```python
from build123d import *

# Parameters (mm, degrees)
F0_W     = 40
F0_H     = 40
F1_DEPTH = 5
F2_R     = 2
F3_DEPTH = 5
F4_R     = 3
F5_DEPTH = 3


with BuildPart() as f1:
    # F0 (on Top) → F1 (new body)
    with BuildSketch(Plane.XY):
        Rectangle(F0_W, F0_H)
    extrude(amount=F1_DEPTH)

    # F2 (on face) → F3 (cut)
    with BuildSketch(Plane.XY.offset(5)):
        with Locations((-12.70971, -8.583505)):
            Circle(F2_R)
        with Locations((-13.331592, 11.416495)):
            Circle(F2_R)
        with Locations((12.668408, 12.357356)):
            Circle(F2_R)
        with Locations((13.29029, -7.642644)):
            Circle(F2_R)
    extrude(amount=-F3_DEPTH, mode=Mode.SUBTRACT)

    # F4 (on face) → F5 (cut)
    with BuildSketch(Plane.XY.offset(5)):
        with Locations((-12.70971, -8.583505)):
            Circle(F4_R)
        with Locations((-13.331592, 11.416495)):
            Circle(F4_R)
        with Locations((12.668408, 12.357356)):
            Circle(F4_R)
        with Locations((13.29029, -7.642644)):
            Circle(F4_R)
    extrude(amount=-F5_DEPTH, mode=Mode.SUBTRACT)


solid = f1.part
```
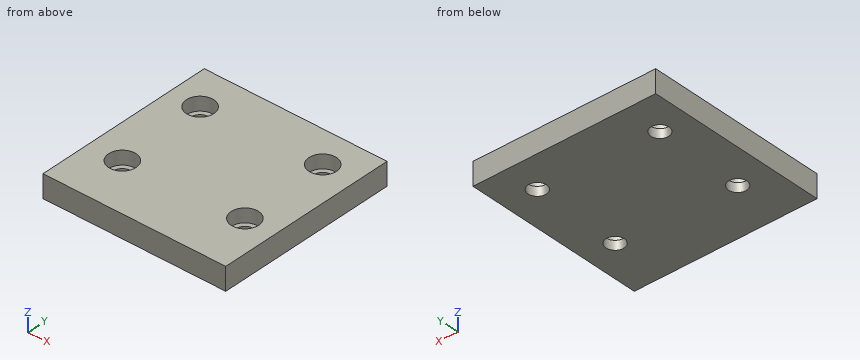
The listing builds one solid part. Answer for the finished solid, in the listing's coordinates (mm). Coordinates: 2 decimals unless noted, no trailing zeros. Loops run counter-clockwise (first coordinate to the right, second up) from the corner with the lowest first, then second, coordinate; pieces in that order, holes last. Notation, with made-up numbers: (57, -13) -> (85, -13) arc R12 cw to (85, -5) -> close; hole circle Ø8 at (61.5, -4). An arc over 180 degrees is marked (long way). Use one line per item in the form item = value. Start each with the question number.
Item 1: The part is cut by section B-B on z = 3. Determine the outline of the cut face in (x, y).
Item 2: A flat-ended cylindrical pin translates along its axis: pin 1 Ø5.5 at (x, y) = (12.67, 12.36) entering from +Z. Find the tip coordinate at first contact, or state that the pin passes through.
Item 3: The part is cut by section D-D on z = 0.55. Determine the outline of the cut face in (x, y), then the cut area to 3 significant figures.
Item 4: The part is cut by section A-A on x = 12. Determine the outline of the cut face in (y, z), then the cut area to 3 significant figures.
Item 5: The part is cut by section C-C on x = -12. Determine the outline of the cut face in (y, z).
Item 6: Consider L1, parallel to Y at x = -11, z = 3.5; L2, parallel to Y at x = 13, z = 0.65; L3, parallel to X at y = -8, z = 2.05. Determine where each line is inside the solid, lowest interval first. Write a range as [from, to].
Answer key:
q1.outline = (-20, -20) -> (20, -20) -> (20, 20) -> (-20, 20) -> close; hole circle Ø6 at (-13.33, 11.42); hole circle Ø6 at (-12.71, -8.58); hole circle Ø6 at (12.67, 12.36); hole circle Ø6 at (13.29, -7.64)
q2.pin_1 = 2
q3.outline = (-20, -20) -> (20, -20) -> (20, 20) -> (-20, 20) -> close; hole circle Ø4 at (-13.33, 11.42); hole circle Ø4 at (-12.71, -8.58); hole circle Ø4 at (12.67, 12.36); hole circle Ø4 at (13.29, -7.64)
q3.area = 1,550 mm2
q4.outline = (-20, 0) -> (-9.17, 0) -> (-9.17, 2) -> (-10.35, 2) -> (-10.35, 5) -> (-20, 5) -> close; (-6.11, 0) -> (10.47, 0) -> (10.47, 2) -> (9.43, 2) -> (9.43, 5) -> (-4.93, 5) -> (-4.93, 2) -> (-6.11, 2) -> close; (14.24, 0) -> (20, 0) -> (20, 5) -> (15.28, 5) -> (15.28, 2) -> (14.24, 2) -> close
q4.area = 153 mm2
q5.outline = (-20, 0) -> (-10.45, 0) -> (-10.45, 2) -> (-11.5, 2) -> (-11.5, 5) -> (-20, 5) -> close; (-6.71, 0) -> (9.92, 0) -> (9.92, 2) -> (8.73, 2) -> (8.73, 5) -> (-5.67, 5) -> (-5.67, 2) -> (-6.71, 2) -> close; (12.91, 0) -> (20, 0) -> (20, 5) -> (14.1, 5) -> (14.1, 2) -> (12.91, 2) -> close
q6.L1 = [-20, -11.05], [-6.12, 9.53], [13.3, 20]
q6.L2 = [-20, -9.62], [-5.66, 10.39], [14.33, 20]
q6.L3 = [-20, -15.65], [-9.77, 10.31], [16.27, 20]
